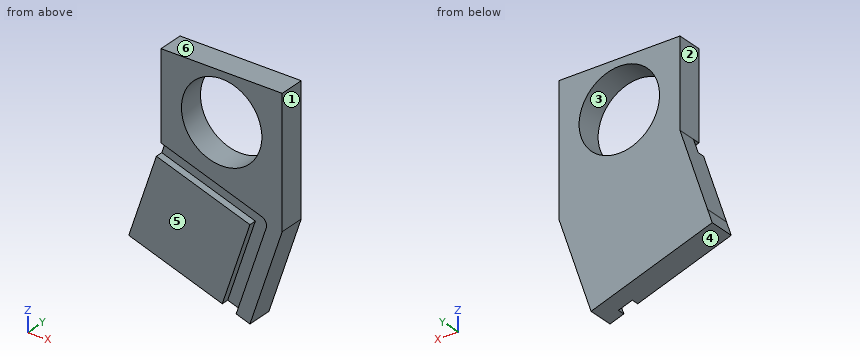
Autodesk Inventor part; units mm, degrees
ref_plane "YZ Plane" through (0, 0, 0) normal (1, 0, 0) x (0, 1, 0)
ref_plane "XZ Plane" through (0, 0, 0) normal (0, 1, 0) x (-1, 0, 0)
ref_plane "XY Plane" through (0, 0, 0) normal (0, 0, 1) x (1, 0, 0)
sketch "Sketch1" plane through (0, 0, 0) normal (0, 1, 0) x (-1, 0, 0)
  line L0 (-8.0312, -19.6194) -> (-8.0312, -0.5694)
  line L1 (-8.0312, -0.5694) -> (-34.5277, -0.5694)
  line L2 (-34.5277, -0.5694) -> (-34.5277, -28.5056)
  line L3 (18.6455, 5.0782) -> (18.6456, 5.0782)
  line L4 (-1.974, -37.6808) -> (-8.0312, -19.6194)
  line L5 (-34.5277, -28.5056) -> (-27.4611, -49.5771)
  line L6 (-1.974, -37.6808) -> (-0.9645, -40.691)
  line L7 (-27.4611, -49.5771) -> (-0.9645, -40.691)
  circle A0 centre (-21.2794, -10.9517) radius 8.7948
  line L8 (-8.0312, -0.5694) -> (-8.0312, -19.6194)
  line L9 (-8.0312, -19.6194) -> (-0.9645, -40.691)
  line L10 (-0.9645, -40.691) -> (-27.4611, -49.5771)
  line L11 (-27.4611, -49.5771) -> (-34.5277, -28.5056)
  line L12 (-34.5277, -28.5056) -> (-34.5277, -0.5694)
  line L13 (-34.5277, -0.5694) -> (-8.0312, -0.5694)
  dimension "d0" = 19.05
  dimension "d1" = 22.225
  dimension "d2" = 27.9469
  dimension "d3" = 26.4965
  dimension "d4" = 17.5895
  dimension "d18" = 13.2483
  dimension "d20" = 161.46
  dimension "d22" = 10.3823
extrude "Extrusion1" add sketch "Sketch1" along normal blind 5.588
sketch "Sketch2" plane through (0, 0, 0) normal (0, -1, 0) x (1, 0, 0)
  line L0 (27.4611, -49.5771) -> (0.9645, -40.691)
  line L1 (31.5175, -27.4959) -> (29.9883, -26.9832)
  line L2 (34.5277, -28.5056) -> (27.4611, -49.5771)
  line L3 (27.4611, -49.5771) -> (0.9645, -40.691)
  line L4 (31.5175, -27.4959) -> (8.0312, -19.6194)
  line L5 (8.0312, -19.6194) -> (7.0136, -22.6537)
  line L6 (7.0136, -22.6537) -> (27.4656, -29.5126)
  line L7 (24.4508, -48.5675) -> (21.4165, -47.5499)
  line L8 (21.4165, -47.5499) -> (27.4656, -29.5126)
  line L9 (29.9883, -26.9831) -> (31.5175, -27.4959)
  line L10 (31.5175, -27.4959) -> (24.4508, -48.5675)
  point P0 (0, 0)
  dimension "d15" = 3.2004
  dimension "d16" = 3.175
  dimension "d17" = 3.2004
extrude "Extrusion2" cut sketch "Sketch2" against normal blind 1.5875
fillet "Fillet1" radius 1.5875 1 edges at (31.5175, 0.7937, -27.4959)
properties part number "Lidar Sensor CAse Piece 1"
CAD build for the part. Positions are in the model's coordinates, mm. Face numbers are marked on the shaded views. A direction names the side the tool comes from. Round coordinates to 2 decimals unless told otherwise and drop trailing zeros. Write each loop counter-clockwise with the first axis right and the second up, starting at its lowest first coordinate (ties: lowest second). Pieces come first, ordered by that corner, then holes. Notation, with made-up numbers: (79.5, 24) -> (94.5, 24) arc R19 ccw to (94.5, 54) -> close; hole circle Ø8 at (57.5, -28). An arc over 180 degrees is marked (long way). Answer in a Markdown table with one row per item. Add a question column.
Item 1: Mould opens along Z. For the marked faces 3, 4, 5 and 6 say: pulls with the +Z half, pulls with the -Z half, needs draft (parallel to the pull), parting line crosses it, or undercut.
Item 2: Drop flat-ended pins along their axis: pin 1 Ø1 at (x, z) = (4.5, -31.5) entering from -Y; pin 2 Ø1 at (x, y) = (21, 2.5) entering from -Z; pin 3 Ø2 at (y, z) = (3.5, -9) entering from -X; pin 4 Ø1 at (y, z) = (4, -37.5) entering from -X. Give the stop position or say it passes through.
Item 3: Drill centre lines: line 1 (Y direction, x = 27.5, z = -36); line 2 (X direction, y = 5.05, z = -11); line 3 (X direction, y = 3.3, z = -4.5). Where is each one in solid material? Low to high. Write a range as from..to.
Item 4: Saw through at C-C, the plane y = 3.2. Write the cut outline in (x, z), then the cut area to 3 significant figures.
Item 5: Which spindle directions (+Z, -Z, +X, -X, +Y, -Y) get a long thin tool onto all of the face, cutting with end or side? Do the marked faces 1 and 2. Say none if no direction does.
Item 6: Saw through at B-B, the plane z = -9.5. Write the cut outline in (x, y).
Item 7: Saw through at A-A, the plane y = 0.9. Count the separate pieces of the cut face and the enclosed holes in it, then the cut area to 3 significant figures.
Item 8: Saw through at D-D, the plane x = 14. Write the cut outline in (y, z), then the cut area to 3 significant figures.
Findings below:
| question | item | result |
|---|---|---|
| 1 | face 3 | undercut |
| 1 | face 4 | pulls with the -Z half |
| 1 | face 5 | needs draft |
| 1 | face 6 | pulls with the +Z half |
| 2 | pin 1 | stops at y = 0 |
| 2 | pin 2 | stops at z = -47.58 |
| 2 | pin 3 | stops at x = 8.03 |
| 2 | pin 4 | stops at x = 1.87 |
| 3 | line 1 | y = 1.59..5.59 |
| 3 | line 2 | x = 8.03..12.48, 30.07..34.53 |
| 3 | line 3 | x = 8.03..15.3, 27.26..34.53 |
| 4 | outline | (0.96, -40.69) -> (27.46, -49.58) -> (34.53, -28.51) -> (34.53, -0.57) -> (8.03, -0.57) -> (8.03, -19.62) -> (1.97, -37.68) -> close; hole circle Ø17.59 at (21.28, -10.95) |
| 4 | area | 1,000 mm^2 |
| 5 | face 1 | +Z, -Z, +X, +Y, -Y |
| 5 | face 2 | +Z, -X, +Y, -Y |
| 6 | outline | (8.03, 0) -> (12.61, 0) -> (12.61, 5.59) -> (8.03, 5.59) -> close; (29.95, 0) -> (34.53, 0) -> (34.53, 5.59) -> (29.95, 5.59) -> close |
| 7 | separate pieces | 2 |
| 7 | enclosed holes | 1 |
| 7 | area | 861 mm^2 |
| 8 | outline | (0, -45.06) -> (5.59, -45.06) -> (5.59, -15.89) -> (0, -15.89) -> (0, -21.62) -> (1.59, -21.62) -> (1.59, -25) -> (0, -25) -> close; (0, -6.02) -> (5.59, -6.02) -> (5.59, -0.57) -> (0, -0.57) -> close |
| 8 | area | 188 mm^2 |
